Here's how the part is built. I have some questions about the finished solid (model axes, mm). A direction names the side the tool comes from. Coordinates: 2 decimals unless noted, no trailing zeros. Loops run counter-clockwise (first coordinate to the right, second up) from the corner with the lowest first, then second, coordinate; pieces in that order, holes last. Notation, with made-up numbers: M 13,69 L 22,69 A25 cw 22,90 Z; hole C -12,84.5 d1. An arc over 180 degrees is marked long. Use one line per item in the form item = value. Start each with the question number.
(1) Will these pins go through, and if not, where does the flat tip stop? P1, Ø1.6, axis at x = -5.8, z = 46.45, coming from the -Y side (1 decimal); P2, Ø2, axis at x = -8.5, z = 18, coming from the -Y side; P3, Ø5, axis at x = -2, z = 56.5, coming from the -Y side.
(2) Imagine slicing it at D-D, the plane y = 11. Please give me the cut outline in (x, z), and give its area (3 significant figures).
(3) Imagine slicing it at A-A, the plane y = 19. Please give me the cut outline in (x, z), and give its area (3 significant figures).
(4) On a 3-axis mill with a long thin cutter (end or side, diameter ignored), from which of +Z, -Z, +X, -X, +Y, -Y can I reach the whole of each face in a straight line? I mean faces 5 (the flat face through (0, 22, 0)), 6 (the cylindrical face through (0.19, 33.23, 56.3)). Say none if no direction works.
(5) Thinking about a two-plate mould opening in Z: for faces 1 (the cylindrical face through (0.17, 7.25, 59.94)), 2 (the flat face through (0, 18, 6)), 3 (the flat face through (0, 18, 56.9)), 4 (the flat face through (0, 22, 62.9)), which applies, +Z half, -Z half, draft (parallel to the pull), parting line (faces both ways), or undercut?
(6) Imagine slicing it at C-C, the plane x = 0. Please give me the cut outline in (y, z), and give its area (3 significant figures).
(7) Imagine slicing it at B-B, the plane z = 46.45. Please give me the cut outline in (x, y), and give its area (3 significant figures).
(8) Please list where these lines run through material, in increasing order: L1, parallel to Z at x = -5.8, y = 35.05; L2, parallel to Z at x = -9, y = 12; L3, parallel to Y at x = -1, z = 45.
Autodesk Inventor part; units mm, degrees
ref_plane "YZ Plane" through (0, 0, 0) normal (1, 0, 0) x (0, 1, 0)
ref_plane "XZ Plane" through (0, 0, 0) normal (0, 1, 0) x (-1, 0, 0)
ref_plane "XY Plane" through (0, 0, 0) normal (0, 0, 1) x (1, 0, 0)
ref_plane "작업 평면1" through (0, 0, 0) normal (0, 0, 1) x (1, 0, 0)
sketch "스케치1" plane through (0, 0, 0) normal (0, 0, 1) x (1, 0, 0)
  circle A0 centre (0, 0) radius 13.8
  circle A1 centre (0, 0) radius 7.2
  circle A2 centre (0, -11) radius 1.2813
  circle A3 centre (-7.7782, -7.7782) radius 1.2813
  circle A4 centre (-11, 0) radius 1.2813
  circle A5 centre (-7.7782, 7.7782) radius 1.2813
  circle A6 centre (0, 11) radius 1.2813
  circle A7 centre (7.7782, 7.7782) radius 1.2813
  circle A8 centre (11, 0) radius 1.2813
  circle A9 centre (7.7782, -7.7782) radius 1.2813
  line L0 (-13.8, 0) -> (-13.8, 13.8)
  line L1 (-13.8, 13.8) -> (13.8, 13.8)
  line L2 (13.8, 13.8) -> (13.8, 0)
  circle A10 centre (0, 0) radius 7.25
  arc A11 (7.2344, 0.4753) -> (13.8, 0) centre (10.5, 0) ccw
  arc A12 (-13.8, 0) -> (-7.2344, 0.4753) centre (-10.5, 0) ccw
  line L3 (7.25, 0) -> (7.2, 0)
  line L4 (-7.2, 0) -> (-7.25, 0)
  circle A13 centre (11, 0) radius 1.35
  circle A14 centre (7.7782, 7.7782) radius 1.35
  circle A15 centre (0, 11) radius 1.35
  circle A16 centre (-7.7782, 7.7782) radius 1.35
  circle A17 centre (-11, 0) radius 1.35
  line L5 (13.8, 13.8) -> (-13.8, 13.8)
  line L6 (-13.8, 13.8) -> (-13.8, 33.8)
  line L7 (-13.8, 33.8) -> (13.8, 33.8)
  line L8 (13.8, 33.8) -> (13.8, 13.8)
  line L9 (3, 33.8) -> (-3, 33.8)
  line L10 (-3, 33.8) -> (-3, 39.8)
  line L11 (-3, 39.8) -> (3, 39.8)
  line L12 (3, 39.8) -> (3, 33.8)
  point P0 (0, 0)
  point P1 (-7.2344, -0.4753)
  point P2 (7.2344, -0.4753)
  dimension "d0" = 14.5
  dimension "d1" = 2.7
  dimension "d2" = 2.7
  dimension "d3" = 2.7
  dimension "d4" = 2.7
  dimension "d5" = 2.7
  dimension "d6" = 20
  dimension "d7" = 6
  dimension "d8" = 6
extrude "돌출1" add sketch "스케치1" along normal blind 6 contours L0 L1 A0 | A0 A11 A10 A12 | A0 L1 L2 | L1 L6 L7 L8 | L10 L11 L12 L7 picked at (-4.6271, 10.5053)
sketch "스케치2" plane through (-3, 39.8, 0) normal (0, 1, 0) x (1, 0, 0)
  circle A0 centre (-5, -3) radius 1.35
  circle A1 centre (11, -3) radius 1.35
  point P0 (3, 0)
  dimension "d11" = 2.7
  dimension "d12" = 2.7
extrude "돌출2" cut sketch "스케치2" against normal blind 20
sketch "스케치3" plane through (0, 0, 6) normal (0, 0, 1) x (1, 0, 0)
  line L0 (-9.35, 33.8) -> (-9.35, 19.8)
  line L1 (-6.65, 33.8) -> (-6.65, 19.8)
  line L2 (15, 15) -> (-15, 15)
  line L3 (6.65, 33.8) -> (6.65, 19.8)
  line L4 (9.35, 33.8) -> (9.35, 19.8)
  line L5 (9.35, 26.8) -> (6.65, 26.8)
  line L6 (-6.65, 26.8) -> (-9.35, 26.8)
  line L7 (10.6, 27.9) -> (5.4, 27.9)
  line L8 (5.4, 27.9) -> (5.4, 25.7)
  line L9 (5.4, 25.7) -> (10.6, 25.7)
  line L10 (10.6, 25.7) -> (10.6, 27.9)
  line L11 (10.6, 27.9) -> (5.4, 25.7) construction
  line L12 (5.4, 27.9) -> (10.6, 25.7) construction
  line L13 (-5.4, 27.9) -> (-10.6, 27.9)
  line L14 (-10.6, 27.9) -> (-10.6, 25.7)
  line L15 (-10.6, 25.7) -> (-5.4, 25.7)
  line L16 (-5.4, 25.7) -> (-5.4, 27.9)
  line L17 (-5.4, 27.9) -> (-10.6, 25.7) construction
  line L18 (-10.6, 27.9) -> (-5.4, 25.7) construction
  point P0 (0, 0)
  point P1 (8, 26.8)
  point P2 (-8, 26.8)
  dimension "d15" = 5.2
  dimension "d16" = 2.2
  dimension "d17" = 5.2
  dimension "d18" = 2.2
extrude "돌출3" cut sketch "스케치3" against normal blind 20
sketch "스케치4" plane through (-3, 39.8, 0) normal (0, 1, 0) x (1, 0, 0)
  line L0 (-2, 0) -> (8, 0)
  line L1 (8, 0) -> (8, -6)
  line L2 (8, -6) -> (-2, -6)
  line L3 (-2, -6) -> (-2, 0)
  line L4 (-2, 0) -> (8, -6) construction
  line L5 (8, 0) -> (-2, -6) construction
  point P0 (3, 0)
  point P1 (3, -3)
  dimension "d21" = 10
  dimension "d22" = 6
extrude "돌출4" add sketch "스케치4" against normal blind 6
sketch "스케치5" plane through (0, 0, 6) normal (0, 0, 1) x (1, 0, 0)
  line L0 (-5, 33.8) -> (-13.8, 33.8)
  line L1 (13.8, 33.8) -> (5, 33.8)
  line L2 (-5, 39.8) -> (-5, 33.8)
  line L3 (-13.8, 33.8) -> (-13.8, 0)
  line L4 (13.8, 0) -> (13.8, 33.8)
  line L5 (-5, 39.8) -> (5, 39.8)
  line L6 (-13.8, 33.8) -> (13.8, 33.8)
  line L7 (13.8, 33.8) -> (13.8, 39.8)
  line L8 (13.8, 39.8) -> (-13.8, 39.8)
  line L9 (-13.8, 39.8) -> (-13.8, 33.8)
  point P0 (0, 0)
  point P1 (5, 39.8)
extrude "돌출5" cut sketch "스케치5" against normal blind 10
sketch "스케치6" plane through (0, 0, 6) normal (0, 0, 1) x (1, 0, 0)
  line L0 (-13.8, 33.8) -> (-13.8, 0)
  line L1 (13.8, 33.8) -> (-13.8, 33.8)
  line L2 (13.8, 0) -> (13.8, 33.8)
  line L3 (-13.8, 33.8) -> (13.8, 33.8)
  line L4 (13.8, 33.8) -> (13.8, 14.8)
  line L5 (13.8, 14.8) -> (-13.8, 14.8)
  line L6 (-13.8, 14.8) -> (-13.8, 33.8)
  point P0 (0, 0)
  point P1 (-13.8, 14.8)
  dimension "d27" = 19
extrude "돌출6" add sketch "스케치6" against normal blind 6
sketch "스케치7" plane through (0, 0, 6) normal (0, 0, 1) x (1, 0, 0)
  line L0 (13.8, 33.8) -> (-13.8, 33.8)
  line L1 (-13.8, 33.8) -> (-13.8, 0)
  arc A0 (-13.8, 0) -> (-7.2344, -0.4753) centre (-10.5, 0) ccw
  line L2 (13.8, 0) -> (13.8, 33.8)
  line L3 (-13.8, 33.8) -> (13.8, 33.8)
  line L4 (13.8, 33.8) -> (13.8, 39.8)
  line L5 (13.8, 39.8) -> (-13.8, 39.8)
  line L6 (-13.8, 39.8) -> (-13.8, 33.8)
  point P0 (0, 0)
  dimension "d30" = 6
extrude "돌출7" add sketch "스케치7" along normal blind 25.45
sketch "스케치8" plane through (0, 0, 6) normal (0, 0, -1) x (-1, 0, 0)
  line L0 (13.8, 39.8) -> (13.8, 33.8)
  line L1 (-13.8, 33.8) -> (13.8, 33.8)
  line L2 (13.8, 39.8) -> (13.8, 33.8)
  line L3 (-13.8, 39.8) -> (13.8, 39.8)
  line L4 (-13.8, 33.8) -> (-13.8, 39.8)
  line L5 (-13.8, 39.8) -> (13.8, 39.8)
  line L6 (-13.8, 39.8) -> (13.8, 39.8)
  line L7 (13.8, 39.8) -> (13.8, 33.8)
  line L8 (13.8, 33.8) -> (-13.8, 33.8)
  line L9 (-13.8, 33.8) -> (-13.8, 39.8)
  point P0 (0, 0)
extrude "돌출8" add sketch "스케치8" along normal blind 6
sketch "스케치9" plane through (-13.8, 39.8, 31.45) normal (0, 1, 0) x (1, 0, 0)
  line L0 (0, 31.45) -> (0, 0)
  line L1 (27.6, 0) -> (0, 0)
  line L2 (27.6, 31.45) -> (27.6, 0)
  line L3 (0, 31.45) -> (27.6, 31.45)
  line L4 (27.6, 25.45) -> (0, 25.45)
  circle A0 centre (8, 15) radius 1.35
  circle A1 centre (19.6, 15) radius 1.35
  point P0 (13.8, 31.45)
  dimension "d35" = 2.7
  dimension "d36" = 2.7
extrude "돌출9" cut sketch "스케치9" against normal blind 6 contours A0 | A1
fillet "모깎기1" radius 2 2 edges at (0, 39.8, 0) (0, 33.8, 6)
mirror "미러1" about plane through (0, 36.8, 31.45) normal (0, 0, 1)
properties part number "foot_right_64" material "PMMA 플라스틱"
Answer:
q1.P1 = through
q1.P2 = 33.8
q1.P3 = 5.71
q2.outline = M -13.8,0 L -1.35,0 L -1.35,6 L -13.8,6 Z; M -13.8,56.9 L -1.35,56.9 L -1.35,62.9 L -13.8,62.9 Z; M 1.35,0 L 13.8,0 L 13.8,6 L 1.35,6 Z; M 1.35,56.9 L 13.8,56.9 L 13.8,62.9 L 1.35,62.9 Z
q2.area = 299 mm²
q3.outline = M -13.8,0 L 13.8,0 L 13.8,6 L -13.8,6 Z; M -13.8,56.9 L 13.8,56.9 L 13.8,62.9 L -13.8,62.9 Z
q3.area = 331 mm²
q4.face_5 = -Z, +X, -X, +Y, -Y
q4.face_6 = +X, -X, -Y
q5.face_1 = draft
q5.face_2 = undercut
q5.face_3 = undercut
q5.face_4 = +Z half
q6.outline = M 7.25,0 L 9.65,0 L 9.65,6 L 7.25,6 Z; M 7.25,56.9 L 9.65,56.9 L 9.65,62.9 L 7.25,62.9 Z; M 12.35,0 L 37.8,0 A2 ccw 39.8,2 L 39.8,60.9 A2 ccw 37.8,62.9 L 12.35,62.9 L 12.35,56.9 L 31.8,56.9 A2 cw 33.8,54.9 L 33.8,8 A2 cw 31.8,6 L 12.35,6 Z
q6.area = 664 mm²
q7.outline = M -13.8,33.8 L -7.15,33.8 L -7.15,39.8 L -13.8,39.8 Z; M -4.45,33.8 L 4.45,33.8 L 4.45,39.8 L -4.45,39.8 Z; M 7.15,33.8 L 13.8,33.8 L 13.8,39.8 L 7.15,39.8 Z
q7.area = 133 mm²
q8.L1 = 0 to 15.1, 17.8 to 45.1, 47.8 to 62.9
q8.L2 = 0 to 6, 56.9 to 62.9
q8.L3 = 33.8 to 39.8
